```python
from build123d import *

# Parameters (mm, degrees)
BOSS_EXTRUDE1_DEPTH = 78


with BuildPart() as part:
    # Sketch1 → Boss-Extrude1 (new body)
    with BuildSketch(Plane.XY):
        with BuildLine():
            Line((-2, 3), (-2, 5.123475383))
            ThreePointArc((-2, 5.123475383), (-3.102418411, -4.541475531), (5.5, 0))
            ThreePointArc((5.5, 0), (4.541475531, 3.102418411), (2, 5.123475383))
            Line((2, 5.123475383), (2, 3))
            Line((2, 3), (-2, 3))
        make_face()
    extrude(amount=BOSS_EXTRUDE1_DEPTH)


solid = part.part
```
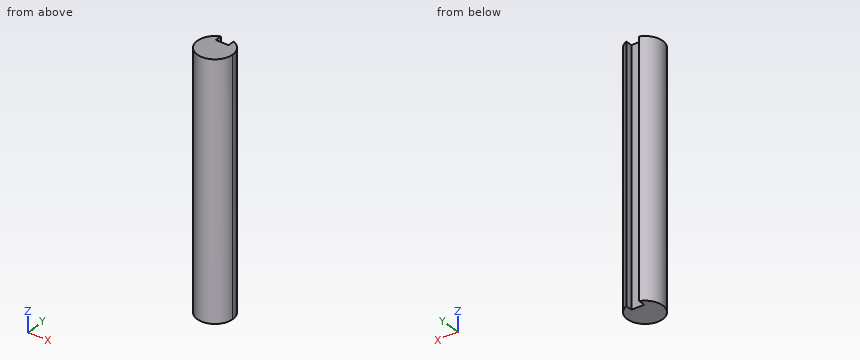
Design review of the part built by this model. Coordinates are the model's own, in mm. Round coordinates to 2 decimals unless told otherwise and drop trailing zeros. Write each loop counter-clockwise with the first axis right and the second up, starting at its lowest first coordinate (ties: lowest second). Pieces come first, ordered by that corner, then holes. Notation, with made-up numbers: (68, 39.25) -> (125, 39.25) arc R17 cw to (125, 48.25) -> close; hole circle Ø4 at (33, -14). An arc over 180 degrees is marked (long way). Write item = value, one per line. Start each with the question number.
1) Take a section at B-B, the plane x = 0. State the section outline as (y, z) points.
2) Clearance check with flat-ended pins moving along their axes: pin 1 (2 mm diameter, centred on x = 0.5, z = 55, fed in from +Y); pin 2 (2.5 mm diameter, centred on y = 3.5, z = 43.5, fed in from -X); pin 3 (1 mm diameter, centred on y = 2.5, z = 34.5, fed in from -X). State where each tip first meets the part, or that it passes through.
3) Take a section at A-A, the plane z = 17.5. State the section outline as (x, y) points, plus the area to 3 significant figures.
4) Take a section at C-C, the plane y = -2.25. State the section outline as (x, z) points, plus the area to 3 significant figures.
5) Wall thickness on probe 1 along X at (y, z) = (4.25, 67.5); probe 2 along X at (y, z) = (0.25, 23); probe 3 along X at (y, z) = (4.75, 43.5): over which ranges is each line inside the solid? List them lowest first. Write a range as from..to.
Results list:
q1.outline = (-5.5, 0) -> (3, 0) -> (3, 78) -> (-5.5, 78) -> close
q2.pin_1 = 3
q2.pin_2 = -5.02
q2.pin_3 = -5.12
q3.outline = (-2, 3) -> (-2, 5.12) arc R5.5 ccw (long way) to (2, 5.12) -> (2, 3) -> close
q3.area = 85.5 mm²
q4.outline = (-5.02, 0) -> (5.02, 0) -> (5.02, 78) -> (-5.02, 78) -> close
q4.area = 783 mm²
q5.probe_1 = -3.49..-2, 2..3.49
q5.probe_2 = -5.49..5.49
q5.probe_3 = -2.77..-2, 2..2.77
